Here's the drawing with two shaded views (mm, measured from the low corner). I have some questions. Round coordinates to 2 decimals unless told otherwise and drop trailing zeros. Loops run counter-clockwise (first coordinate to the right, second up) from the corner with the lowest first, then second, coordinate; pieces in that order, holes last. Notation, with made-up numbers: (62, 72.25) - (103, 72.25) arc R26 cw to (103, 103.25) - close; hole circle Ø3 at (25.5, -6). An arc over 180 degrees is marked (long way). Use one line per item in the form item = value.
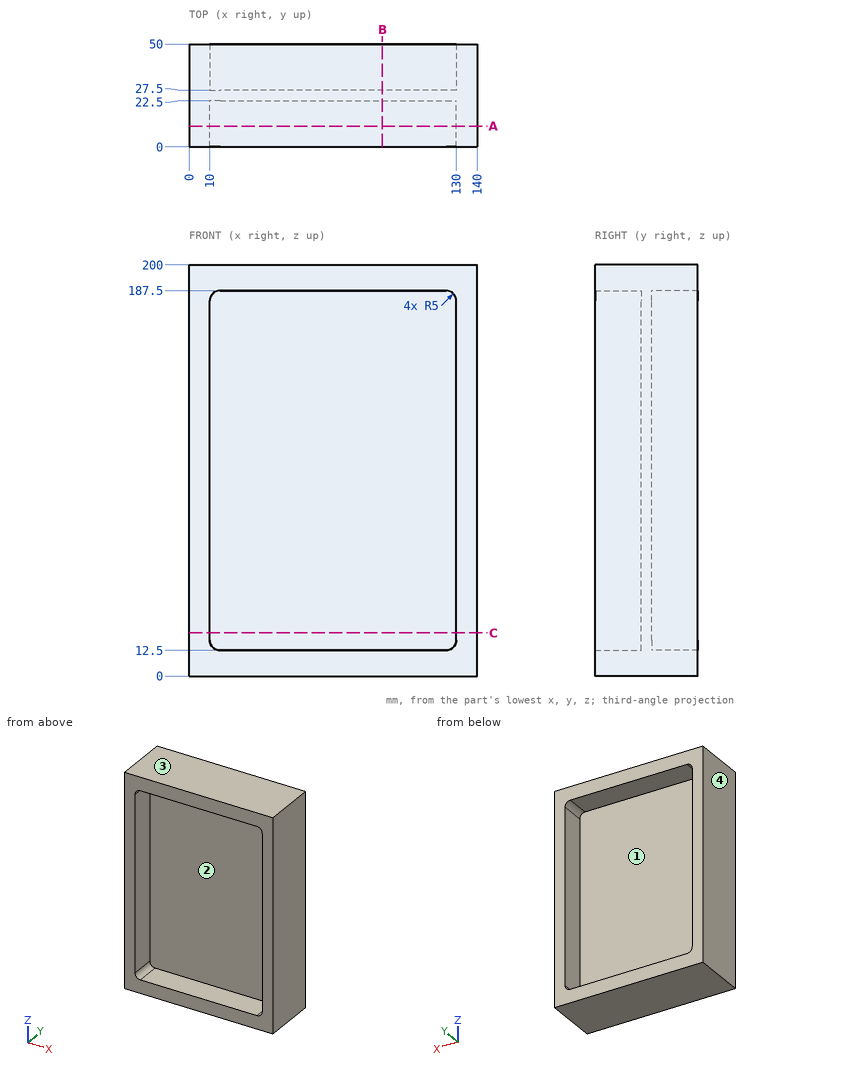
1. If we section it at B-B, the plane x = 94: Write out the boundary of the cut face in (y, z), plus the area to 4 significant figures.
Solution:
outline = (0, 0) - (50, 0) - (50, 12.5) - (27.5, 12.5) - (27.5, 187.5) - (50, 187.5) - (50, 200) - (0, 200) - (0, 187.5) - (22.5, 187.5) - (22.5, 12.5) - (0, 12.5) - close
area = 2,125 mm^2
2. If we section it at A-A, the plane y = 10: Write out the boundary of the cut face in (x, z).
Solution:
outline = (0, 0) - (140, 0) - (140, 200) - (0, 200) - close; hole (10, 17.5) arc R5 ccw to (15, 12.5) - (125, 12.5) arc R5 ccw to (130, 17.5) - (130, 182.5) arc R5 ccw to (125, 187.5) - (15, 187.5) arc R5 ccw to (10, 182.5) - close
3. We'd pull the mould along X, two halves only. Please class the marked faces 1, 2, 3 and 4: +X half, -X half, draft (parallel to the pull), parting line (faces both ways), or undercut.
Solution:
face_1 = undercut
face_2 = undercut
face_3 = draft
face_4 = -X half
4. For P1, Ø3, axis at x = 66.5, z = 177.5, coming from the +Y side; P2, Ø1, axis at x = 65, z = 116.5, coming from the -Y side, each with a flat end and sliding along its axis, tell me the tip position at first contact or that it passes through.
Solution:
P1 = 27.5
P2 = 22.5
5. If we section it at C-C, the plane z = 21: Write out the boundary of the cut face in (x, y).
Solution:
outline = (0, 0) - (10, 0) - (10, 22.5) - (130, 22.5) - (130, 0) - (140, 0) - (140, 50) - (130, 50) - (130, 27.5) - (10, 27.5) - (10, 50) - (0, 50) - close
6. Please list where these lines run through material, in increasing order: line 1 along Z through (x, y) = (53, 22); line 2 along X through (y, z) = (39, 152); line 3 along Y through (x, z) = (112.5, 145).
Solution:
line_1 = 0 to 12.5, 187.5 to 200
line_2 = 0 to 10, 130 to 140
line_3 = 22.5 to 27.5
